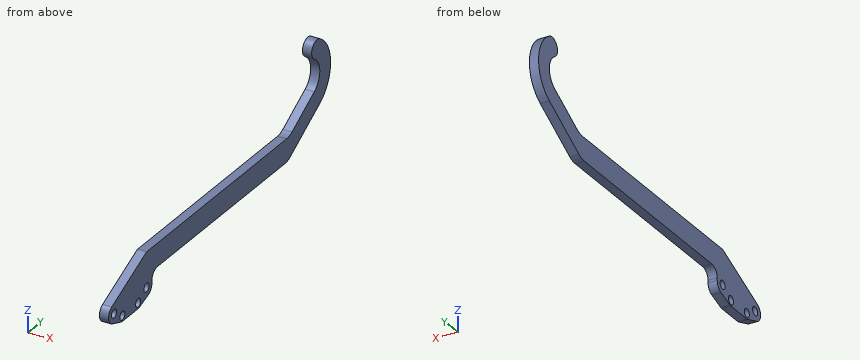
from build123d import *

# Parameters (mm, degrees)
BOSS_EXTRUDE1_DEPTH = 3.175
FILLET1_R           = 12.7
SKETCH2_R           = 2.9845
CUT_EXTRUDE1_DEPTH  = 248.533087061
FILLET2_R           = 6.35


with BuildPart() as part:
    # Sketch1 → Boss-Extrude1 (new, symmetric)
    with BuildSketch(Plane(origin=(0, 0, 0), x_dir=(0, 0, -1), z_dir=(1, 0, 0))):
        with BuildLine():
            Line((-8.731303996, -21.648910397), (-26.9875, 19.05))
            Line((-26.9875, 19.05), (-26.9875, 186.759204744))
            Line((-26.9875, 186.759204744), (-43.811945986, 215.9))
            ThreePointArc((-43.811945986, 215.9), (-54.810468614, 222.25), (-65.808991242, 215.9))
            ThreePointArc((-65.808991242, 215.9), (-74.483252556, 213.575738686), (-76.80751387, 222.25))
            ThreePointArc((-76.80751387, 222.25), (-54.810468614, 234.95), (-32.813423357, 222.25))
            Line((-32.813423357, 222.25), (-11.1125, 184.662898174))
            Line((-11.1125, 184.662898174), (-11.1125, 25.4))
            Line((-11.1125, 25.4), (-2.9375, 25.4))
            ThreePointArc((-2.9375, 25.4), (0.751942089, 24.218221848), (3.068123689, 21.112761283))
            Line((3.068123689, 21.112761283), (6.691014805, 10.56489959))
            ThreePointArc((6.691014805, 10.56489959), (6.852071397, 9.929208286), (6.90625, 9.275673789))
            Line((6.90625, 9.275673789), (6.90625, -9.275673789))
            ThreePointArc((6.90625, -9.275673789), (6.852071397, -9.929208286), (6.691014805, -10.56489959))
            Line((6.691014805, -10.56489959), (3.068123689, -21.112761283))
            ThreePointArc((3.068123689, -21.112761283), (-2.649262487, -25.393454827), (-8.731303996, -21.648910397))
        make_face()
    extrude(amount=BOSS_EXTRUDE1_DEPTH, both=True)

    # Fillet1
    fillet1_edges = [part.edges().sort_by_distance(p)[0] for p in [
        (0, 186.759204744, 26.9875),
        (0, 184.662898174, 11.1125),
    ]]
    fillet(fillet1_edges, radius=FILLET1_R)

    # Sketch2 → Cut-Extrude1 (cut, through all)
    with BuildSketch(Plane(origin=(3.175, 0, 0), x_dir=(0, 0, -1), z_dir=(1, 0, 0))):
        with Locations((-2.9375, 19.05)):
            Circle(SKETCH2_R)
        with Locations((2.9375, -9.275673789)):
            Circle(SKETCH2_R)
        with Locations((-2.9375, -19.05)):
            Circle(SKETCH2_R)
        with Locations((2.9375, 9.275673789)):
            Circle(SKETCH2_R)
    extrude(amount=-CUT_EXTRUDE1_DEPTH, mode=Mode.SUBTRACT)

    # Fillet2
    fillet2_edges = [part.edges().sort_by_distance(p)[0] for p in [
        (0, 25.4, 11.1125),
    ]]
    fillet(fillet2_edges, radius=FILLET2_R)


solid = part.part
Source: CAD feature listing. Evaluate the final solid. Frame: model axes, mm. Give positions to 0.01 mm unless a question says otherwise; leave off trailing zeros. Write each loop counter-clockwise with the first axis right and the second up, starting at its lowest first coordinate (ties: lowest second). Pieces come first, ordered by that corner, then holes. Notation, with made-up numbers: M 66,83.5 L 94,83.5 A33 ccw 94,121.5 Z; hole C -27,14.5 d1. An arc over 180 degrees is marked long. Answer as a JSON object with one key per item and string values.
Q1. Contact query for flat-ended pins moving along their axis: P1, Ø3, axis at x = -1, y = 132.5, coming from the -Z side; P2, Ø3.5, axis at y = -9.28, z = -2.94, coming from the -X side; P3, Ø1.5, axis at x = 0, z = 64.5, coming from the -Y side; P4, Ø2, axis at x = -0.5, z = 4, coming from the +Y side. Output: stop coordinate, or through.
Geometry check:
{"P1": "stops at z = 11.11", "P2": "passes through", "P3": "stops at y = 216.78", "P4": "stops at y = 25.4"}
Q2. Cut plane C-C, the plane z = 19.5. Return the cut outline in (x, y) (3 decimals), then the cut area to 3 significant figures.
Geometry check:
{"outline": "M -3.175,2.358 L 3.175,2.358 L 3.175,199.19 L -3.175,199.19 Z", "area": "1,250 mm^2"}
Q3. Ray query, line 1 along Y through (x, z) = (-2.25, 3); line 2 along Z through (x, y) = (1.5, 86); line 3 along Y through (x, z) = (1.5, 1). Return the intervals inside material, ascending.
Geometry check:
{"line 1": "y = -25.4 to -22.03, -16.07 to 16.07, 22.03 to 25.4", "line 2": "z = 11.11 to 26.99", "line 3": "y = -25.1 to -21.32, -16.78 to 16.78, 21.32 to 25.1"}
Q4. Cut plane B-B, the plane y = 110. Return the cut outline in (x, z) (1 decimal).
Geometry check:
{"outline": "M -3.2,11.1 L 3.2,11.1 L 3.2,27 L -3.2,27 Z"}
Q5. Cut plane A-A, the plane x = 1.25. Count the separate pieces of the cut face and the enclosed holes in it, then the cut area to 3 significant figures.
Geometry check:
{"separate pieces": "1", "enclosed holes": "4", "area": "4,690 mm^2"}
